Geometry: final body of the model. Coordinates: model frame, mm. Round coordinates to 2 decimals unless told otherwise and drop trailing zeros. Loops run counter-clockwise (first coordinate to the right, second up) from the corner with the lowest first, then second, coordinate; pieces in that order, holes last. Notation, with made-up numbers: (89, 45.25) - (136, 45.25) arc R16 cw to (136, 76.25) - close; hole circle Ø7 at (-10.5, -24). An arc over 180 degrees is marked (long way). Answer as a JSON object with one key per item and string values. Group by question number.
Item 1: Line query: line 1 (Z direction, x = 0, y = 1.7); line 2 (Y direction, x = -18, z = 7); line 3 (X direction, y = 1.65, z = 4.5). Output: solid intervals per line, ascending.
Item 2: Section C-C (x = -23.5). Return the cut outline in (y, z).
Item 3: Section A-A (x = -0.5). Return the cut outline in (y, z).
Item 4: Section B-B (z = 0). Return the cut outline in (x, y), plus the area to 3 significant figures.
Item 5: First-contact query: pin 1 (1.5 mm diameter, centred on x = -24.5, z = 0, fed in from +Y). Flat tip, straight axial feed; report the tip coordinate or a pass-through.
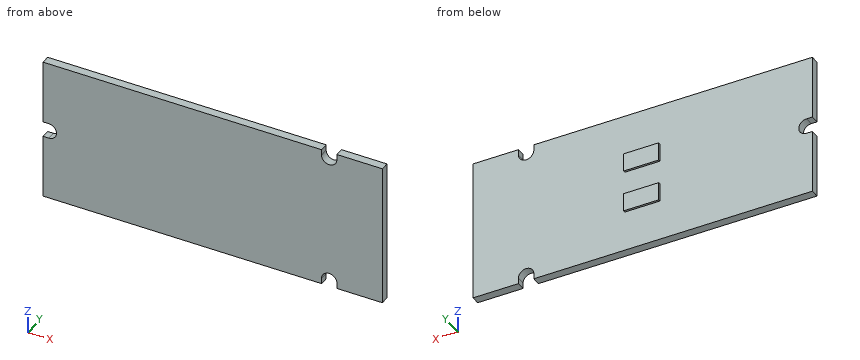
```python
from build123d import *

# Parameters (mm, degrees)
BOSS_EXTRUDE1_DEPTH = 1.6
SKETCH2_W           = 6.6
SKETCH2_H           = 3.45
BOSS_EXTRUDE2_DEPTH = 0.4


with BuildPart() as part:
    # Sketch1 → Boss-Extrude1 (new body)
    with BuildSketch(Plane(origin=(0, 0, 0), x_dir=(1, 0, 0), z_dir=(0, 1, 0))):
        with BuildLine():
            Line((31.95, -13.45), (23.4, -13.45))
            Line((23.4, -13.45), (23.4, -12.375))
            ThreePointArc((23.4, -12.375), (21.95, -10.925), (20.5, -12.375))
            Line((20.5, -12.375), (20.5, -13.45))
            Line((20.5, -13.45), (-31.95, -13.45))
            Line((-31.95, -13.45), (-31.95, -1.45))
            Line((-31.95, -1.45), (-30.85, -1.45))
            ThreePointArc((-30.85, -1.45), (-29.4, 0), (-30.85, 1.45))
            Line((-30.85, 1.45), (-31.95, 1.45))
            Line((-31.95, 1.45), (-31.95, 13.45))
            Line((-31.95, 13.45), (20.5, 13.45))
            Line((20.5, 13.45), (20.5, 12.375))
            ThreePointArc((20.5, 12.375), (21.95, 10.925), (23.4, 12.375))
            Line((23.4, 12.375), (23.4, 13.45))
            Line((23.4, 13.45), (31.95, 13.45))
            Line((31.95, 13.45), (31.95, -13.45))
        make_face()
    extrude(amount=BOSS_EXTRUDE1_DEPTH)

    # Sketch2 → Boss-Extrude2 (add)
    with BuildSketch(Plane(origin=(0, 1.6, 0), x_dir=(1, 0, 0), z_dir=(0, 1, 0))):
        with Locations((0.05, 4.075)):
            Rectangle(SKETCH2_W, SKETCH2_H)
        with Locations((0.05, -3.925)):
            Rectangle(SKETCH2_W, SKETCH2_H)
    extrude(amount=BOSS_EXTRUDE2_DEPTH)


solid = part.part
```
Values:
{
 "1": {"line 1": "z = -5.8 to -2.35, 2.2 to 5.65", "line 2": "y = 0 to 1.6", "line 3": "x = -3.25 to 3.35"},
 "2": {"outline": "(0, -13.45) - (1.6, -13.45) - (1.6, 13.45) - (0, 13.45) - close"},
 "3": {"outline": "(0, -13.45) - (1.6, -13.45) - (1.6, -5.8) - (2, -5.8) - (2, -2.35) - (1.6, -2.35) - (1.6, 2.2) - (2, 2.2) - (2, 5.65) - (1.6, 5.65) - (1.6, 13.45) - (0, 13.45) - close"},
 "4": {"outline": "(-29.4, 0) - (31.95, 0) - (31.95, 1.6) - (-29.4, 1.6) - close", "area": "98.2 mm^2"},
 "5": {"pin 1": "stops at y = 1.6"}
}
